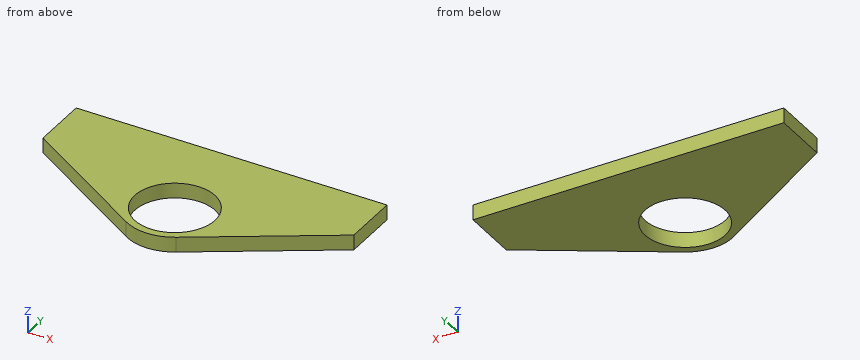
from build123d import *

# Parameters (mm, degrees)
SKETCH_1_R             = 10.65
SM_BASE_FLANGE_1_DEPTH = 4


# Sheet-metal steps are written as plain solids
with BuildPart() as part:
    # Sketch 1 → Базовая кромка1 (new body)
    with BuildSketch(Plane.XY):
        with BuildLine():
            Line((0, 0), (-34.594362709, -21.407039383))
            ThreePointArc((-34.594362709, -21.407039383), (-41.250833524, -23.3), (-47.907304338, -21.407039383))
            Line((-47.907304338, -21.407039383), (-82.501667048, 0))
            Line((-82.501667048, 0), (-82.501667048, 15))
            Line((-82.501667048, 15), (0, 15))
            Line((0, 15), (0, 0))
        make_face()
        with Locations((-41.250833524, -10.65)):
            Circle(SKETCH_1_R, mode=Mode.SUBTRACT)
    extrude(amount=-SM_BASE_FLANGE_1_DEPTH)


solid = part.part
Model file for the job. Use its own axes, mm. Coordinates: 2 decimals unless noted, no trailing zeros. Write each loop counter-clockwise with the first axis right and the second up, starting at its lowest first coordinate (ties: lowest second). Pieces come first, ordered by that corner, then holes. Notation, with made-up numbers: (-15.5, 82.25) - (-1.5, 82.25) arc R17 cw to (-1.5, 99.25) - close; hole circle Ø4 at (78, -6). An arc over 180 degrees is marked (long way). Write each question's results on one line, items separated by ' | '. Start each with the question number.
1) Probe line 1 along Y through (x, z) = (-50.5, -1.9); line 2 along X through (y, z) = (-4, -0.95); line 3 along Y through (x, z) = (-35, -1.95). List the from-to ranges inside material, lowest first. Write a range as from..to.
2) Flat gauge pins, fed straight in: P1, Ø2, axis at y = -10, z = -2, coming from the -X side; P2, Ø2, axis at y = -4, z = -1, coming from the -X side; P3, Ø1.5, axis at y = -14, z = -2.5, coming from the +X side. Where does each tip first touch, or does it go through?
3) Cut at B-B (y = -9). Write the cut outline in (x, z).
4) Cut at A-A (z = -3.3). Write the cut outline in (x, y), then the cut area to 3 significant figures.
5) Cut at C-C (x = -46.5). Write the cut outline in (y, z), then the cut area to 3 significant figures.
6) Cut at D-D (x = -18). Write the cut outline in (y, z), then the cut area to 3 significant figures.
Returned:
1) line 1: -19.8..-15.93, -5.37..15 | line 2: -76.04..-49.57, -32.93..-6.46 | line 3: -21.65..-19.27, -2.03..15
2) P1: x = -67.96 | P2: x = -77.65 | P3: x = -21.41
3) outline: (-67.96, -4) - (-51.77, -4) - (-51.77, 0) - (-67.96, 0) - close; (-30.73, -4) - (-14.54, -4) - (-14.54, 0) - (-30.73, 0) - close
4) outline: (-82.5, 0) - (-47.91, -21.41) arc R12.65 ccw to (-34.59, -21.41) - (0, 0) - (0, 15) - (-82.5, 15) - close; hole circle Ø21.3 at (-41.25, -10.65) | area: 1,920 mm^2
5) outline: (-22.16, -4) - (-19.92, -4) - (-19.92, 0) - (-22.16, 0) - close; (-1.38, -4) - (15, -4) - (15, 0) - (-1.38, 0) - close | area: 74.5 mm^2
6) outline: (-11.14, -4) - (15, -4) - (15, 0) - (-11.14, 0) - close | area: 105 mm^2
